```python
from build123d import *

# Parameters (mm, degrees)
SKETCH_R   = 8.05
SKETCH_R_2 = 1.6
PAD_DEPTH  = 5
FILLET_R   = 3


with BuildPart() as part:
    # Sketch → Pad (new body)
    with BuildSketch(Plane.XY):
        Polygon((15, 16), (15, -16), (15, -23.2), (-31, -23.2), (-31, -16), (-31, 16), (-31, 23.2), (15, 23.2), align=None)
        Circle(SKETCH_R, mode=Mode.SUBTRACT)
        with Locations((-24, 9)):
            Circle(SKETCH_R_2, mode=Mode.SUBTRACT)
        with Locations((-24, -9)):
            Circle(SKETCH_R_2, mode=Mode.SUBTRACT)
        with Locations((9, -9)):
            Circle(SKETCH_R_2, mode=Mode.SUBTRACT)
        with Locations((9, 9)):
            Circle(SKETCH_R_2, mode=Mode.SUBTRACT)
        with Locations((0, 20.5)):
            Circle(SKETCH_R_2, mode=Mode.SUBTRACT)
        with Locations((0, -20.5)):
            Circle(SKETCH_R_2, mode=Mode.SUBTRACT)
        with Locations((-21, 19.6)):
            Circle(SKETCH_R_2, mode=Mode.SUBTRACT)
        with Locations((5, 19.6)):
            Circle(SKETCH_R_2, mode=Mode.SUBTRACT)
        with Locations((-21, -19.6)):
            Circle(SKETCH_R_2, mode=Mode.SUBTRACT)
        with Locations((5, -19.6)):
            Circle(SKETCH_R_2, mode=Mode.SUBTRACT)
    extrude(amount=PAD_DEPTH)

    # Fillet
    fillet_edges = [part.edges().sort_by_distance(p)[0] for p in [
        (-31, -23.2, 2.5),
        (-31, 23.2, 2.5),
        (15, 23.2, 2.5),
        (15, -23.2, 2.5),
    ]]
    fillet(fillet_edges, radius=FILLET_R)


solid = part.part
```
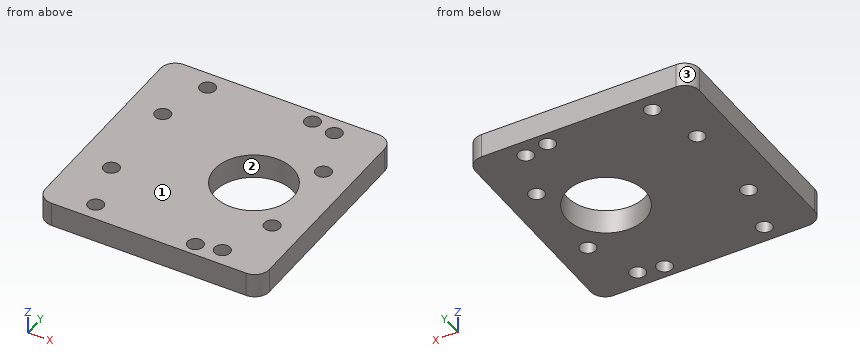
Verification items for the finished model (mm, model axes). Face numbers are marked on the shaded views. Give positions to 0.01 mm unless a question says otherwise; leave off trailing zeros. Loops run counter-clockwise (first coordinate to the right, second up) from the corner with the lowest first, then second, coordinate; pieces in that order, holes last. Notation, with made-up numbers: M 23.5,22.25 L 55.5,22.25 A31 ccw 55.5,58.25 Z; hole C 26.25,82.25 d8. An arc over 180 degrees is marked long. One line per question, with ' | ' between items.
Item 1: Depth check by flat-ended pin: P1, Ø2, axis at x = -12, y = 2, coming from the -Z side. Enter the tip coordinate at first touch or a pass-through.
Completed:
P1: stops at z = 0
Item 2: Section check B-B, the plane x = -21. Record the cut outline in (y, z), plus the area to 3 significant figures.
Completed:
outline: M -23.2,0 L -21.2,0 L -21.2,5 L -23.2,5 Z; M -18,0 L 18,0 L 18,5 L -18,5 Z; M 21.2,0 L 23.2,0 L 23.2,5 L 21.2,5 Z | area: 200 mm^2
Item 3: Draft check along X on the marked faces 1, 2 and 3. Enter one of: +X half, -X half, draft (parallel to the pull), parting line (faces both ways), or undercut.
Completed:
face 1: draft | face 2: undercut | face 3: -X half
Item 4: Section check D-D, the plane x = 0. Record the cut outline in (y, z).
Completed:
outline: M -23.2,0 L -22.1,0 L -22.1,5 L -23.2,5 Z; M -18.9,0 L -8.05,0 L -8.05,5 L -18.9,5 Z; M 8.05,0 L 18.9,0 L 18.9,5 L 8.05,5 Z; M 22.1,0 L 23.2,0 L 23.2,5 L 22.1,5 Z
Item 5: Thickness scan on line 1 (Y direction, x = 9, z = 2.6); line 2 (Y direction, x = 0, z = 1.85); line 3 (Y direction, x = -21.5, z = 3.5). Record the ranges inside material, lowest first. Write a range as [from, to].
Completed:
line 1: y = [-23.2, -10.6], [-7.4, 7.4], [10.6, 23.2] | line 2: y = [-23.2, -22.1], [-18.9, -8.05], [8.05, 18.9], [22.1, 23.2] | line 3: y = [-23.2, -21.12], [-18.08, 18.08], [21.12, 23.2]
Item 6: Section check C-C, the plane z = 1.45. State how many separate pieces and enclosed holes the cut face has, plus the area to 3 significant figures.
Completed:
separate pieces: 1 | enclosed holes: 11 | area: 1,840 mm^2
Item 7: Section check A-A, the plane y = 0. Record the cut outline in (x, z).
Completed:
outline: M -31,0 L -8.05,0 L -8.05,5 L -31,5 Z; M 8.05,0 L 15,0 L 15,5 L 8.05,5 Z
